Build history of the part. All positions in model axes, mm. Face numbers are marked on the shaded views. A direction names the side the tool comes from. Give positions to 0.01 mm unless a question says otherwise; leave off trailing zeros. Order: outer loops, then holes, each group sorted by start corner. A loop starts at its lowest first (then second) coordinate and runs counter-clockwise, first axis right, second up. Notation, with made-up numbers: (57, 53.25) - (87, 53.25) arc R21 cw to (87, 60.25) - close; hole circle Ø11 at (-22.5, 59.5). An arc over 180 degrees is marked (long way). Answer in a Markdown table with one row per item.
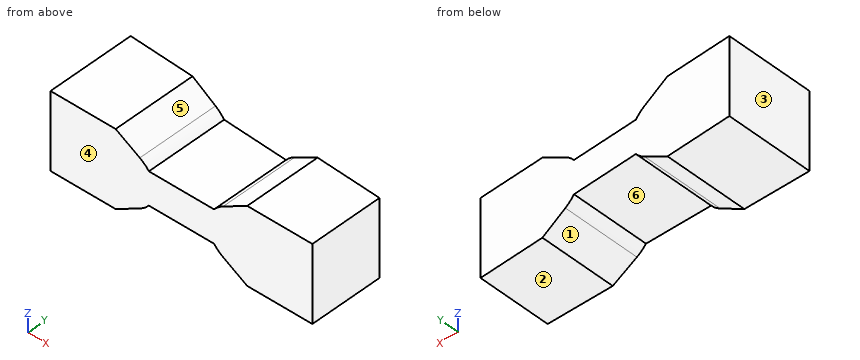
```python
from build123d import *

# Parameters (mm, degrees)
BOSS_EXTRUDE1_DEPTH     = 8
BOSS_EXTRUDE1_2_DEPTH   = 8
BOSS_EXTRUDE2_DEPTH     = 8
CUT_EXTRUDE2_DEPTH      = 15.891142801
CUT_EXTRUDE2_DEPTH_BACK = 15.891142801


with BuildPart() as part:
    # Sketch2 → Boss-Extrude1 (new body)
    with BuildSketch(Plane(origin=(0, 0, 0), x_dir=(1, 0, 0), z_dir=(0, 1, 0))):
        with BuildLine():
            Line((-6.062177826, 3.5), (-12.062177826, 3.5))
            Line((-12.062177826, 3.5), (-12.062177826, -3.5))
            Line((-12.062177826, -3.5), (-6.062177826, -3.5))
            Line((-6.062177826, -3.5), (-3.834419723, -2.213803259))
            ThreePointArc((-3.834419723, -2.213803259), (-3.384272952, -1.895404124), (-3, -1.5))
            Line((-3, -1.5), (-3, 1.5))
            ThreePointArc((-3, 1.5), (-3.384272952, 1.895404124), (-3.834419723, 2.213803259))
            Line((-3.834419723, 2.213803259), (-6.062177826, 3.5))
        make_face()
    extrude(amount=BOSS_EXTRUDE1_DEPTH)



with BuildPart() as body_2:
    # Sketch2 → Boss-Extrude1 2 (new body)
    with BuildSketch(Plane(origin=(0, 0, 0), x_dir=(1, 0, 0), z_dir=(0, 1, 0))):
        with BuildLine():
            Line((3.834419723, 2.213803259), (6.062177826, 3.5))
            Line((6.062177826, 3.5), (12.062177826, 3.5))
            Line((12.062177826, 3.5), (12.062177826, -3.5))
            Line((12.062177826, -3.5), (6.062177826, -3.5))
            Line((6.062177826, -3.5), (3.834419723, -2.213803259))
            ThreePointArc((3.834419723, -2.213803259), (3.384272952, -1.895404124), (3, -1.5))
            Line((3, -1.5), (3, 1.5))
            ThreePointArc((3, 1.5), (3.384272952, 1.895404124), (3.834419723, 2.213803259))
        make_face()
    extrude(amount=BOSS_EXTRUDE1_2_DEPTH)


with BuildPart() as part_1:
    add(part.part)

    add(body_2.part)  # Boss-Extrude2 merges body 2
    # Sketch1 → Boss-Extrude2 (add)
    with BuildSketch(Plane(origin=(0, 0, 0), x_dir=(1, 0, 0), z_dir=(0, 1, 0))):
        with BuildLine():
            Line((3, -1.5), (-3, -1.5))
            ThreePointArc((-3, -1.5), (-3.898777162, -2.249912014), (-5.016117889, -2.598793246))
            ThreePointArc((-5.016117889, -2.598793246), (-5.630991226, -2.399814505), (-5.894085249, -1.809523648))
            Line((-5.894085249, -1.809523648), (-5.894085249, 1.809523648))
            ThreePointArc((-5.894085249, 1.809523648), (-5.630991226, 2.399814505), (-5.016117889, 2.598793246))
            ThreePointArc((-5.016117889, 2.598793246), (-3.898777162, 2.249912014), (-3, 1.5))
            Line((-3, 1.5), (3, 1.5))
            ThreePointArc((3, 1.5), (3.898777162, 2.249912014), (5.016117889, 2.598793246))
            ThreePointArc((5.016117889, 2.598793246), (5.630991226, 2.399814505), (5.894085249, 1.809523648))
            Line((5.894085249, 1.809523648), (5.894085249, -1.809523648))
            ThreePointArc((5.894085249, -1.809523648), (5.630991226, -2.399814505), (5.016117889, -2.598793246))
            ThreePointArc((5.016117889, -2.598793246), (3.898777162, -2.249912014), (3, -1.5))
        make_face()
    extrude(amount=BOSS_EXTRUDE2_DEPTH)

    # Sketch4 → Cut-Extrude2 (cut, two sides: drawn at the far end of the back side and taken through both)
    with BuildSketch(Plane.XY.offset(-CUT_EXTRUDE2_DEPTH_BACK)):
        Polygon((12.062177826, 8), (12.062177826, 6.7), (-12.062177826, 8), align=None)
    extrude(amount=CUT_EXTRUDE2_DEPTH + CUT_EXTRUDE2_DEPTH_BACK, mode=Mode.SUBTRACT)


solid = part_1.part
```
1. Drop flat-ended pins along their axis: P1, Ø3, axis at x = 2.5, y = 2, coming from the +Z side; P2, Ø3, axis at x = -2, y = 4.5, coming from the +Z side; P3, Ø1, axis at x = 3, y = 2, coming from the -Z side. Give the stop position or say it passes through.
Check result:
| item | result |
|---|---|
| P1 | stops at z = 2.31 |
| P2 | stops at z = 1.99 |
| P3 | stops at z = -1.99 |
2. Cut at B-B on x = -2.25. Write the cut outline in (y, z), and give its area (3 significant figures).
Check result:
| item | result |
|---|---|
| outline | (0, -1.5) - (7.47, -1.5) - (7.47, 1.5) - (0, 1.5) - close |
| area | 22.4 mm² |
3. Two-plate mould, pull along X, no slides. Class the marked faces 1, 2 and 3: +X half, -X half, draft (parallel to the pull), parting line (faces both ways), or undercut.
Check result:
| item | result |
|---|---|
| face 1 | undercut |
| face 2 | draft |
| face 3 | -X half |
4. Cut at A-A on y = 3. Write the cut outline in (x, z), and give its area (3 significant figures).
Check result:
| item | result |
|---|---|
| outline | (-12.06, -3.5) - (-6.06, -3.5) - (-3.83, -2.21) arc R3 ccw to (-3, -1.5) - (3, -1.5) arc R3 ccw to (3.83, -2.21) - (6.06, -3.5) - (12.06, -3.5) - (12.06, 3.5) - (6.06, 3.5) - (3.83, 2.21) arc R3 ccw to (3, 1.5) - (-3, 1.5) arc R3 ccw to (-3.83, 2.21) - (-6.06, 3.5) - (-12.06, 3.5) - close |
| area | 134 mm² |
5. Probe line 1 (Z direction, x = -2, y = 1.25); line 2 (X direction, y = 4.5, z = -3); line 3 (Y direction, x = -6, z = 1.5). List the from-to ranges inside material, lowest first.
Check result:
| item | result |
|---|---|
| line 1 | z = -1.5 to 1.5 |
| line 2 | x = -12.06 to -5.2, 5.2 to 12.06 |
| line 3 | y = 0 to 7.67 |
6. Which spindle directions (+Z, -Z, +X, -X, +Y, -Y) get a long thin tool onto all of the face, cutting with end or side? Do the marked faces 4, 5 and 6. Say none if no direction does.
Check result:
| item | result |
|---|---|
| face 4 | +Z, -Z, +X, -X, -Y |
| face 5 | +Z, +Y, -Y |
| face 6 | -Z, +Y, -Y |
7. Cut at C-C on z = 0.5. Write the cut outline in (x, y), and give its area (3 significant figures).
Check result:
| item | result |
|---|---|
| outline | (-12.06, 0) - (12.06, 0) - (12.06, 6.7) - (-12.06, 8) - close |
| area | 177 mm² |
